Can you work these out from the model? Positions are in its coordinate system, mm. A direction names the side the tool comes from. Round coordinates to 2 decimals unless told otherwise and drop trailing zeros. Loops run counter-clockwise (first coordinate to the right, second up) from the corner with the lowest first, then second, coordinate; pieces in that order, holes last. Notation, with made-up numbers: (65.25, 79.25) -> (73.25, 79.25) arc R23 cw to (73.25, 97.25) -> close; hole circle Ø9 at (54, 62). An arc over 180 degrees is marked (long way). Write each question's results on one line, items separated by ' | '.
from build123d import *

# Parameters (mm, degrees)
CROQUIS1_R              = 122.5
SALIENTE_EXTRUIR1_DEPTH = 10
CROQUIS4_R              = 2.6
CROQUIS5_R              = 99.75
CROQUIS5_R_2            = 90
SALIENTE_EXTRUIR3_DEPTH = 10
REDONDEO1_R             = 5
CROQUIS7_R              = 7.4
CROQUIS7_R_2            = 3.3
CROQUIS7_R_3            = 6.4
CORTAR_EXTRUIR1_DEPTH   = 175.391800266


with BuildPart() as part:
    # Croquis1 → Saliente-Extruir1 (new body)
    with BuildSketch(Plane(origin=(0, 0, 0), x_dir=(1, 0, 0), z_dir=(0, 1, 0))):
        with Locations(Location((0, 0, 0), (0, 0, 270))):
            Circle(CROQUIS1_R)
    extrude(amount=SALIENTE_EXTRUIR1_DEPTH)

    # Cortar-Barrer1: sweep along a path in Croquis3
    with BuildLine(Plane(origin=(0, 10, 0), x_dir=(1, 0, 0), z_dir=(0, 1, 0))) as cortar_barrer1_path:
        CenterArc((0, 0), 110, 0, 360)
    # Croquis4 → Cortar-Barrer1 (sweep, cut)
    with BuildSketch(Plane.XY):
        with Locations((-110, 10)):
            Circle(CROQUIS4_R)
    sweep(path=cortar_barrer1_path.line, mode=Mode.SUBTRACT)

    # Croquis5 → Saliente-Extruir3 (add)
    with BuildSketch(Plane(origin=(0, 10, 0), x_dir=(1, 0, 0), z_dir=(0, 1, 0))):
        with Locations(Location((0, 0, 0), (0, 0, 270))):
            Circle(CROQUIS5_R)
        with Locations(Location((0, 0, 0), (0, 0, 270))):
            Circle(CROQUIS5_R_2, mode=Mode.SUBTRACT)
    extrude(amount=SALIENTE_EXTRUIR3_DEPTH)

    # Redondeo1
    redondeo1_edges = [part.edges().sort_by_distance(p)[0] for p in [
        (0, 0, -122.5),
    ]]
    fillet(redondeo1_edges, radius=REDONDEO1_R)

    # Croquis7 → Cortar-Extruir1 (cut, through all)
    with BuildSketch(Plane.XZ):
        with Locations(Location((0, 20, 0), (0, 0, 270))):
            Circle(CROQUIS7_R)
        with Locations(Location((0, -20, 0), (0, 0, 270))):
            Circle(CROQUIS7_R_2)
        with Locations(Location((70, 0, 0), (0, 0, 270))):
            Circle(CROQUIS7_R_3)
        with Locations(Location((-70, 0, 0), (0, 0, 270))):
            Circle(CROQUIS7_R_3)
    extrude(amount=-CORTAR_EXTRUIR1_DEPTH, mode=Mode.SUBTRACT)


solid = part.part
1. If we section it at B-B (z = 0): List the corners of the cut face in (x, y) for me.
Final values:
outline: (-122.5, 5) arc R5 ccw to (-117.5, 0) -> (-76.4, 0) -> (-76.4, 10) -> (-90, 10) -> (-90, 20) -> (-99.75, 20) -> (-99.75, 10) -> (-107.4, 10) arc R2.6 cw to (-112.6, 10) -> (-122.5, 10) -> close; (-63.6, 0) -> (63.6, 0) -> (63.6, 10) -> (-63.6, 10) -> close; (76.4, 0) -> (117.5, 0) arc R5 ccw to (122.5, 5) -> (122.5, 10) -> (112.6, 10) arc R2.6 cw to (107.4, 10) -> (99.75, 10) -> (99.75, 20) -> (90, 20) -> (90, 10) -> (76.4, 10) -> close
2. If we section it at A-A (x = 0): List the corners of the cut face in (y, z) for me.
Final values:
outline: (0, -117.5) arc R5 ccw to (5, -122.5) -> (10, -122.5) -> (10, -112.6) arc R2.6 cw to (10, -107.4) -> (10, -99.75) -> (20, -99.75) -> (20, -90) -> (10, -90) -> (10, -23.3) -> (0, -23.3) -> close; (0, -16.7) -> (10, -16.7) -> (10, 12.6) -> (0, 12.6) -> close; (0, 27.4) -> (10, 27.4) -> (10, 90) -> (20, 90) -> (20, 99.75) -> (10, 99.75) -> (10, 107.4) arc R2.6 cw to (10, 112.6) -> (10, 122.5) -> (5, 122.5) arc R5 ccw to (0, 117.5) -> close
3. If we section it at C-C (y = 16.75): List the corners of the cut face in (x, z) for me, then the cut area to 3 significant figures.
Final values:
outline: circle Ø199.5 at (0, 0); hole circle Ø180 at (0, 0) | area: 5,810 mm2
4. Please list where these lines run through material, in increasing order: line 1 (X direction, y = 5.25, z = 0); line 2 (X direction, y = 8, z = 0); line 3 (X direction, y = 9.75, z = -32). Write a range as from..to.
Final values:
line 1: -122.5..-76.4, -63.6..63.6, 76.4..122.5 | line 2: -122.5..-111.66, -108.34..-76.4, -63.6..63.6, 76.4..108.34, 111.66..122.5 | line 3: -118.25..-107.94, -102.53..102.53, 107.94..118.25
5. We'd pull the mould along Z, two halves only. Please class faces 1 (the face through (76.346, 4.93, 0.833)), 2 (the face through (-119.587, 7.465, -26.556)), 3 (the face through (89, 20, -15)), 4 (the face through (1, 10, -1)): pulls with the +Z half, pulls with the -Z half, needs draft (parallel to the pull), parting line crosses it, or undercut.
Final values:
face 1: undercut | face 2: parting line crosses it | face 3: needs draft | face 4: undercut
6. On a 3-axis mill with a long thin cutter (end or side, diameter ignored), from which of +Z, -Z, +X, -X, +Y, -Y can I reach the whole of each face in a straight line? I mean faces 5 (the face through (-1.26, 4.93, -23.05)), 6 (the face through (-97.38, 14.93, -21.62)). Say none if no direction works.
Final values:
face 5: +Y, -Y | face 6: +Y
7. Will these pins go through, and if not, where does the flat tip stop? pin 1 (12 mm diameter, centred on y = 15.5, z = -12, fed in from -X); pin 2 (3 mm diameter, centred on x = -65.5, y = 13, fed in from -Z); pin 3 (1.5 mm diameter, centred on y = 5.5, z = 62.5, fed in from +X).
Final values:
pin 1: x = -122.12 | pin 2: z = -76.51 | pin 3: x = 105.8
